Design review of the part shown in the three views and the two pictorial views. Dimensions are in mm from the part's minimum x, y and z. A direction names the side the tool comes from. Coordinates: 2 decimals unless noted, no trailing zeros. Loops run counter-clockwise (first coordinate to the right, second up) from the corner with the lowest first, then second, coordinate; pieces in that order, holes last. Notation, with made-up numbers: M 12.5,28 L 40.5,28 A19 cw 40.5,61 Z; hole C -3,79 d10. An arc over 180 degrees is marked long. Put each result on its own line as item: value. Start each with the question number.
(1) Take a section at C-C, the plane z = 65. Give the boundary of the cut face in (x, y) (1 decimal).
(2) Clearance check with flat-ended pins moving along their axes: pin 1 (6 mm diameter, centred on x = 42.5, z = 27.5, fed in from -Y); pin 2 (6 mm diameter, centred on y = 11, z = 70, fed in from +X); pin 3 (12 mm diameter, centred on y = 10, z = 29.5, fed in from +X) (1 decimal). State where each tip first meets the part, or that it passes through.
(3) For the marked faces 1 and 2, list the 3-axis set-ups (+Z, -Z, +X, -X, +Y, -Y) from which the entire face can be reached by the end or side of a thin tool; tool diameter is ignored.
(4) Take a section at B-B, the plane x = 52. Give the boundary of the cut face in (y, z) (1 decimal).
(5) Take a section at A-A, the plane y = 14.25. Give the boundary of the cut face in (x, z) (1 decimal), then the cut area to 3 significant figures.
(6) Take a section at D-D, the plane z = 98. Give the boundary of the cut face in (x, y).
(7) For probe 1 along Y at (x, z) = (36, 99); probe 2 along X at (y, z) = (1, 37) (1 decimal); probe 3 along X at (y, z) = (4.5, 70.5), list the stretches that pass through material, from the lowest coordinate up. Write a range as [from, to].
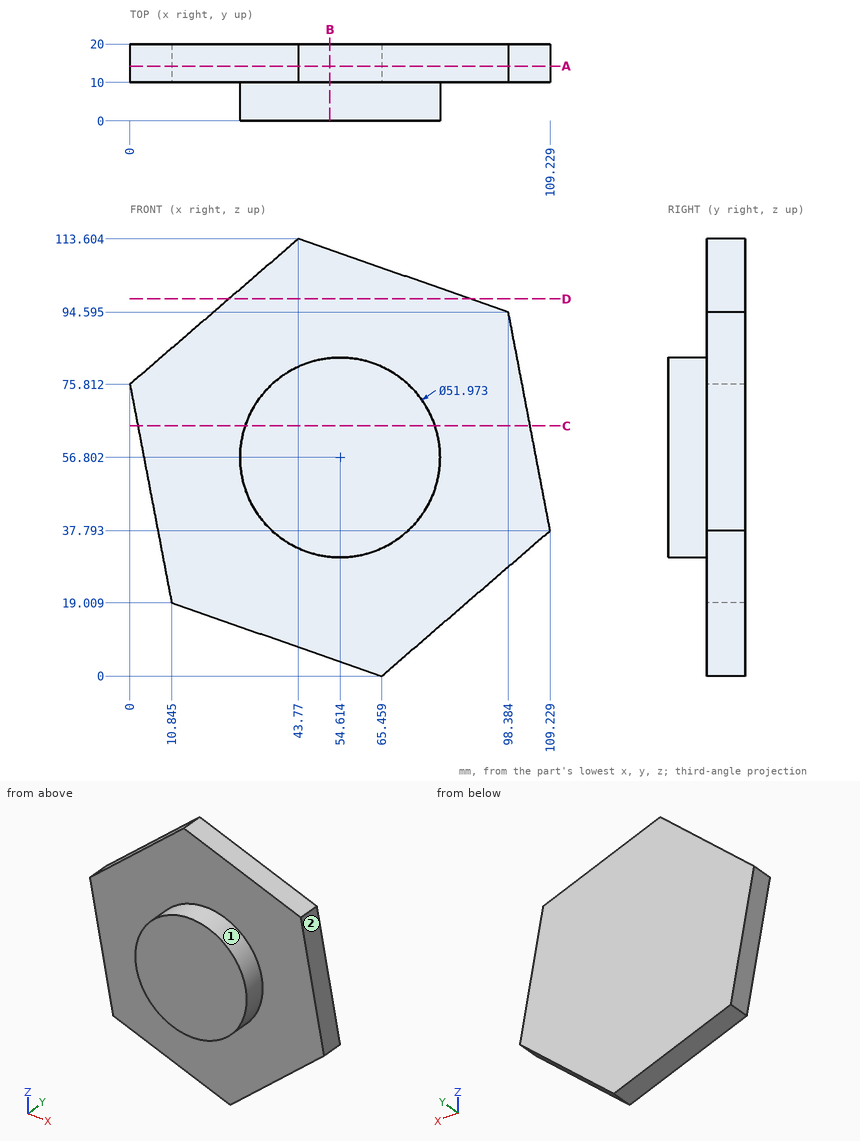
Computed values:
1. outline: M 2.1,10 L 30,10 L 30,0 L 79.3,0 L 79.3,10 L 104,10 L 104,20 L 2.1,20 Z
2. pin 1: stops at y = 10
2. pin 2: stops at x = 103.65
2. pin 3: stops at x = 106.6
3. face 1: -Y
3. face 2: +Z, +X, +Y, -Y
4. outline: M 0,30.9 L 10,30.9 L 10,4.7 L 20,4.7 L 20,110.7 L 10,110.7 L 10,82.7 L 0,82.7 Z
5. outline: M 0,75.8 L 10.8,19 L 65.5,0 L 109.2,37.8 L 98.4,94.6 L 43.8,113.6 Z
5. area: 8,690 mm^2
6. outline: M 25.7,10 L 88.6,10 L 88.6,20 L 25.7,20 Z
7. probe 1: y = [10, 20]
7. probe 2: x = [37.8, 71.4]
7. probe 3: x = [32.53, 76.7]
